from build123d import *

# Parameters (mm, degrees)
SKETCH1_R           = 12.7
SKETCH1_R_2         = 7.5
BOSS_EXTRUDE1_DEPTH = 9.525
FILLET1_R           = 6
SKETCH6_R           = 1.665
CUT_EXTRUDE1_DEPTH  = 123.168257963


with BuildPart() as part:
    # Sketch1 → Boss-Extrude1 (new body)
    with BuildSketch(Plane.XY):
        with BuildLine():
            Line((9, -32), (72.5, -32))
            Line((72.5, -32), (72.5, -25.154302825))
            Line((72.5, -25.154302825), (79.665584639, -25.154302825))
            Line((79.665584639, -25.154302825), (92.440326559, -25.154302825))
            ThreePointArc((92.440326559, -25.154302825), (117.517477972, -0.077151413), (92.440326559, 25))
            Line((92.440326559, 25), (77.7, 25))
            Line((77.7, 25), (0, 25))
            ThreePointArc((0, 25), (-24.382533763, 5.521960459), (-10.771150987, -22.560636215))
            Line((-10.771150987, -22.560636215), (9, -32))
        make_face()
        with Locations(Location((0, 0, 0), (0, 0, 180))):
            Circle(SKETCH1_R, mode=Mode.SUBTRACT)
        with Locations(Location((77.7, 0, 0), (0, 0, 180))):
            Circle(SKETCH1_R_2, mode=Mode.SUBTRACT)
    extrude(amount=BOSS_EXTRUDE1_DEPTH)

    # Fillet1
    fillet1_edges = [part.edges().sort_by_distance(p)[0] for p in [
        (72.5, -25.154302825, 4.7625),
    ]]
    fillet(fillet1_edges, radius=FILLET1_R)

    # Sketch6 → Cut-Extrude1 (cut, through all)
    with BuildSketch(Plane.XY.offset(9.525)):
        with Locations((71.513283589, -14.673233797)):
            Circle(SKETCH6_R)
        with Locations((65.006745214, 5.474046027)):
            Circle(SKETCH6_R)
        with Locations((84.003798538, 14.623316108)):
            Circle(SKETCH6_R)
        with Locations((90.43821159, -5.368599676)):
            Circle(SKETCH6_R)
    extrude(amount=-CUT_EXTRUDE1_DEPTH, mode=Mode.SUBTRACT)


solid = part.part
Part model, mm, in its own coordinate system. A direction names the side the tool comes from. Give positions to 0.01 mm unless a question says otherwise; leave off trailing zeros. Order: outer loops, then holes, each group sorted by start corner. A loop starts at its lowest first (then second) coordinate and runs counter-clockwise, first axis right, second up. Notation, with made-up numbers: (-29, 63) -> (-9, 63) arc R22 cw to (-9, 84) -> close; hole circle Ø2 at (-25.75, -21.75). An arc over 180 degrees is marked (long way). Use one line per item in the form item = value.
(1) Pull direction Y, two halves, no side cores. Call faces 3 (the face through (88.775, -5.295, 4.829)), 4 (the face through (40, -32, 5)), 5 (the face through (-24.274, 5.981, 4.696)), 6 (the face through (-5.86, 11.267, 4.696)): +Y half, -Y half, draft (parallel to the pull), parting line (faces both ways), or undercut.
Solution:
face_3 = undercut
face_4 = -Y half
face_5 = parting line
face_6 = undercut
(2) Saw through at B-B (x = 81). Write the cut outline in (y, z) (3 decimals).
Solution:
outline = (-25.154, 0) -> (-6.735, 0) -> (-6.735, 9.525) -> (-25.154, 9.525) -> close; (6.735, 0) -> (25, 0) -> (25, 9.525) -> (6.735, 9.525) -> close
(3) Tool access for faces 1 (the face through (85, -25.154, 5)), 2 (the face through (117.51, -0.63, 4.7)): list every direction of +Z, -Z, +X, -X, +Y, -Y with a clear straight run to the whole face (end or side of a thin tool).
Solution:
face_1 = +Z, -Z, +X, -Y
face_2 = +Z, -Z, +X
(4) Saw through at A-A (y = 2.5). Write the cut outline in (x, z) (1 decimal).
Solution:
outline = (-24.9, 0) -> (-12.5, 0) -> (-12.5, 9.5) -> (-24.9, 9.5) -> close; (12.5, 0) -> (70.6, 0) -> (70.6, 9.5) -> (12.5, 9.5) -> close; (84.8, 0) -> (117.4, 0) -> (117.4, 9.5) -> (84.8, 9.5) -> close
(5) Flat gauge pins, fed straight in: P1, Ø5, axis at x = 86.5, z = 7, coming from the -Y side; P2, Ø0.9, axis at y = -31.5, z = 7, coming from the +X side; P3, Ø5, axis at y = -22.5, z = 1, coming from the -X side. Where does each tip first touch, or does it go through?
Solution:
P1 = -25.15
P2 = 72.5
P3 = -15
(6) Saw through at C-C (y = -9). Write the cut outline in (x, z) (3 decimals), then the cut area to 3 significant figures.
Solution:
outline = (-23.324, 0) -> (-8.96, 0) -> (-8.96, 9.525) -> (-23.324, 9.525) -> close; (8.96, 0) -> (115.876, 0) -> (115.876, 9.525) -> (8.96, 9.525) -> close
area = 1,160 mm²
(7) Saw through at D-D (z = 7.25). Write the cut outline in (x, y) (3 decimals), then the cut area to 3 significant figures.
Solution:
outline = (-10.771, -22.561) -> (9, -32) -> (72.5, -32) -> (72.5, -31.154) arc R6 cw to (78.5, -25.154) -> (92.44, -25.154) arc R25.077 ccw to (92.44, 25) -> (0, 25) arc R25 ccw to start; hole circle Ø25.4 at (0, 0); hole circle Ø3.33 at (65.007, 5.474); hole circle Ø3.33 at (71.513, -14.673); hole circle Ø15 at (77.7, 0); hole circle Ø3.33 at (84.004, 14.623); hole circle Ø3.33 at (90.438, -5.369)
area = 6,380 mm²
(8) Drill centre lines: line 1 (X direction, y = -4.5, z = 6.75); line 2 (X direction, y = -5.5, z = 4.25); line 3 (Y direction, x = 9, z = 2.25). Where is each one in solid material? Low to high. Write a range as from..to.
Solution:
line_1 = -24.59..-11.88, 11.88..71.7, 83.7..89.02, 91.86..117.12
line_2 = -24.39..-11.45, 11.45..72.6, 82.8..88.78, 92.1..116.92
line_3 = -32..-8.96, 8.96..25
